For this review, take the finished solid that the model builds, in its own axes (mm). A direction names the side the tool comes from. Coordinates: 2 decimals unless noted, no trailing zeros. Order: outer loops, then holes, each group sorted by start corner. A loop starts at its lowest first (then second) coordinate and runs counter-clockwise, first axis right, second up. Notation, with made-up numbers: (25.25, 54) -> (60.25, 54) arc R32 ccw to (60.25, 80) -> close; hole circle Ø7 at (23.25, -14). An arc over 180 degrees is marked (long way). Write item = value, one per line. Start each with the question number.
1) Consider section B-B on y = 4. Give the boundary of the cut face in (x, z), and give its area (3 significant figures).
2) Wall thickness on probe 1 along Y at (x, z) = (-0.6, 1.9); probe 2 along Y at (x, z) = (0.15, -0.9); probe 3 along X at (y, z) = (19.5, 0.4): over which ranges is each line inside the solid? List them lowest first. Write a range as [from, to].
3) Consider section C-C on x = 2.15. Give the boundary of the cut face in (y, z), and give its area (3 significant figures).
4) Machinability: for faces 1 (the face through (0.6, 21, -1.3)), 2 (the face through (0.616, 20.014, -1.088)), which of the approach directions +Z, -Z, +X, -X, +Y, -Y give a long, thin tool a straight path to every point of the face, cutting with its end or side? Answer none if there is none.
5) Consider section D-D on x = -2.1. Give the boundary of the cut face in (y, z).
6) Insertion check: pin 1 Ø1.5 at (x, y) = (2, 18.5) entering from -Z; pin 2 Ø1.5 at (x, y) = (1.5, 3.5) entering from -Z; pin 3 Ø3 at (x, y) = (-1, 5) entering from -Z. Each pin has a flat end and moves straight along its axis. Give the tip position at first contact, or say it passes through.
7) Consider section A-A on z = 0. Give the boundary of the cut face in (x, y), and give its area (4 significant figures).
8) Draft analysis for pull direction X (two halves, no side actions). For faces 3 (the face through (1.5, 9.13, -0.07)), 4 (the face through (1.2, 18, 1.2)), 5 (the face through (1.25, 20, 0)), state which applies: +X half, -X half, draft (parallel to the pull), parting line (faces both ways), or undercut.
Autodesk Inventor part; units mm, degrees
ref_plane "YZ Plane" through (0, 0, 0) normal (1, 0, 0) x (0, 1, 0)
ref_plane "XZ Plane" through (0, 0, 0) normal (0, 1, 0) x (-1, 0, 0)
ref_plane "XY Plane" through (0, 0, 0) normal (0, 0, 1) x (1, 0, 0)
sketch "Sketch1" plane through (0, 0, 0) normal (0, 1, 0) x (-1, 0, 0)
  circle A0 centre (0, 0) radius 1.5
  dimension "d0" = 3
extrude "Extrusion1" add sketch "Sketch1" along normal blind 18
sketch "Sketch2" plane through (0, 18, 0) normal (0, 1, 0) x (1, 0, 0)
  circle A0 centre (0, 0) radius 1.5
  circle A1 centre (0, 0) radius 2.75
  dimension "d3" = 5.5
extrude "Extrusion2" add sketch "Sketch2" along normal blind 3 contours A0 | A1
sketch "Sketch3" plane through (0, 21, 0) normal (0, 1, 0) x (1, 0, 0)
  circle A0 centre (0, 0) radius 2.75
  line L0 (0, 1.4434) -> (1.25, 0.7217)
  line L1 (1.25, 0.7217) -> (1.25, -0.7217)
  line L2 (1.25, -0.7217) -> (0, -1.4434)
  line L3 (0, -1.4434) -> (-1.25, -0.7217)
  line L4 (-1.25, -0.7217) -> (-1.25, 0.7217)
  line L5 (-1.25, 0.7217) -> (0, 1.4434)
  dimension "d6" = 2.5
extrude "Extrusion3" cut sketch "Sketch3" against normal blind 2 contours L0 L1 L2 L3 L4 L5
thread "Thread1"
chamfer "Chamfer1" distance 0.5 angle 45 1 edges at (1.5, 0, 0)
properties part number "M3x18SHCS" material "Stainless Steel"
Answer sheet:
q1.outline = circle Ø3 at (0, 0)
q1.area = 7.07 mm2
q2.probe_1 = [18, 21]
q2.probe_2 = [0, 19]
q2.probe_3 = [-2.72, -1.25], [1.25, 2.72]
q3.outline = (18, -1.71) -> (21, -1.71) -> (21, 1.71) -> (18, 1.71) -> close
q3.area = 10.3 mm2
q4.face_1 = +Z, -Z, +X, -X, +Y
q4.face_2 = +Y
q5.outline = (18, -1.78) -> (21, -1.78) -> (21, 1.78) -> (18, 1.78) -> close
q6.pin_1 = -2.45
q6.pin_2 = -1.3
q6.pin_3 = -1.5
q7.outline = (-2.75, 18) -> (-1.5, 18) -> (-1.5, 0.5) -> (-1, 0) -> (1, 0) -> (1.5, 0.5) -> (1.5, 18) -> (2.75, 18) -> (2.75, 21) -> (1.25, 21) -> (1.25, 19) -> (-1.25, 19) -> (-1.25, 21) -> (-2.75, 21) -> close
q7.area = 65.25 mm2
q8.face_3 = parting line
q8.face_4 = draft
q8.face_5 = undercut
